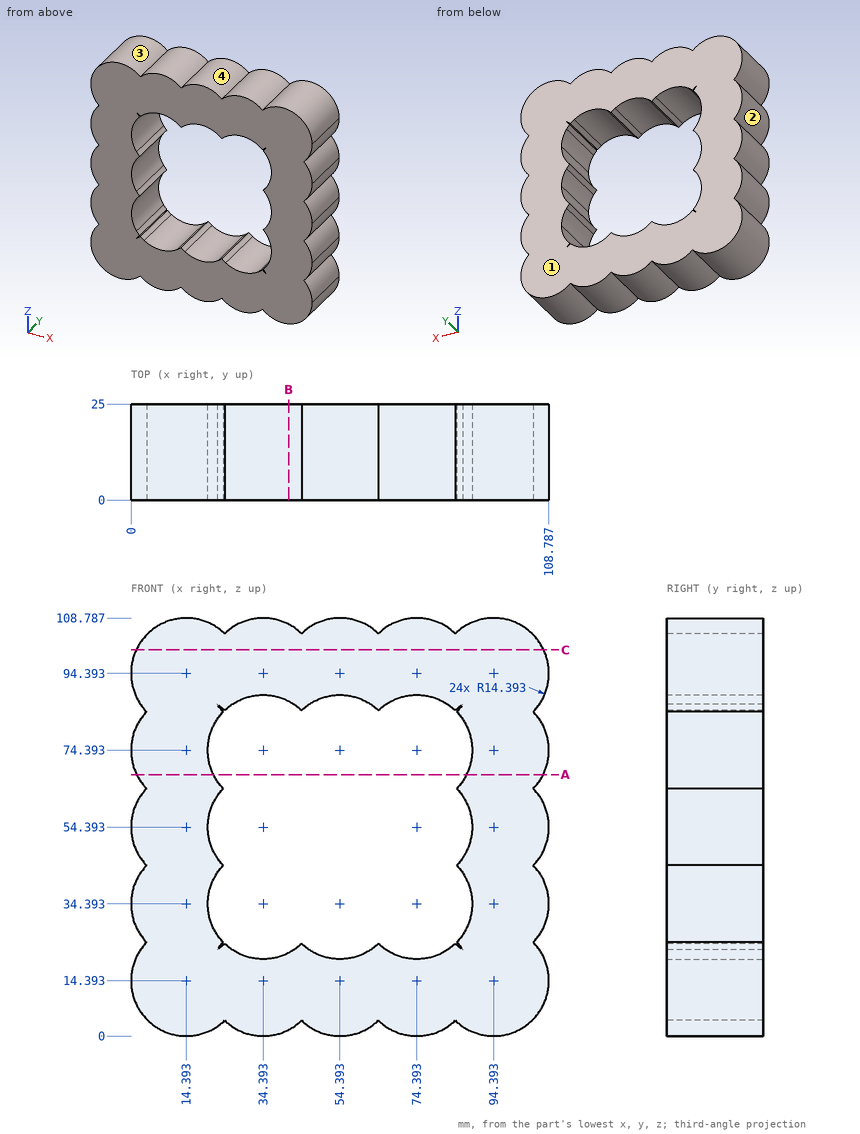
Source: three-view drawing plus pictorial views. Frame: mm from the lowest corner of the part. Give positions to 0.01 mm unless a question says otherwise; leave off trailing zeros. Write each loop counter-clockwise with the first axis right and the second up, starting at its lowest first coordinate (ties: lowest second). Pieces come first, ordered by that corner, then holes. Notation, with made-up numbers: (56.25, 68.5) -> (63.25, 68.5) arc R32 ccw to (63.25, 101.5) -> close; hole circle Ø8 at (-7, 42.5). An arc over 180 degrees is marked (long way). Answer in a Markdown table with one row per item.
(1) Draft query along Z for the marked faces 1, 2, 3 and 4. Return one class per face: +Z half, -Z half, draft (parallel to the pull), parting line (faces both ways), or undercut.
Answers below:
| item | result |
|---|---|
| face 1 | draft |
| face 2 | undercut |
| face 3 | undercut |
| face 4 | +Z half |
(2) Section query B-B on x = 41. Return loops of the section in (y, z), then the cut area to 4 significant figures.
Answers below:
| item | result |
|---|---|
| outline | (0, 1.61) -> (25, 1.61) -> (25, 21.61) -> (0, 21.61) -> close; (0, 87.18) -> (25, 87.18) -> (25, 107.18) -> (0, 107.18) -> close |
| area | 1,000 mm^2 |
(3) Section query A-A on z = 68. Return loops of the section in (x, y), then the cut area to 4 significant figures.
Answers below:
| item | result |
|---|---|
| outline | (1.5, 0) -> (21.5, 0) -> (21.5, 25) -> (1.5, 25) -> close; (87.29, 0) -> (107.29, 0) -> (107.29, 25) -> (87.29, 25) -> close |
| area | 1,000 mm^2 |
(4) Pin query (flat end, axial travel): pin 1 (6 mm diameter, centred on y = 8.5, z = 24, fed in from +X); pin 2 (5 mm diameter, centred on x = 94, y = 6.5, fed in from -Z); pin 3 (2 mm diameter, centred on x = 65.5, y = 6, fed in from -Z); pin 4 (3 mm diameter, centred on y = 8.5, z = 11.5, fed in from +X). Return the tip coordinate at first contact, or that it passes through.
Answers below:
| item | result |
|---|---|
| pin 1 | x = 107.18 |
| pin 2 | z = 0 |
| pin 3 | z = 2.36 |
| pin 4 | x = 108.72 |
(5) Section query C-C on z = 100.5. Return loops of the section in (x, y), then the cut area to 3 significant figures.
Answers below:
| item | result |
|---|---|
| outline | (1.36, 0) -> (107.43, 0) -> (107.43, 25) -> (1.36, 25) -> close |
| area | 2,650 mm^2 |
(6) Ray query, line 1 along Z through (x, y) = (86, 13) (1 decimal); line 2 along X through (y, z) = (23, 87.5) (1 decimal); line 3 along X through (y, z) = (17.5, 25). Return the intervals inside material, ascending. Write a range as [from, to].
Answers below:
| item | result |
|---|---|
| line 1 | [2.7, 22.7], [22.9, 25.9], [42.9, 45.9], [62.9, 65.9], [82.9, 85.9], [86.1, 106.1] |
| line 2 | [1.8, 28.4], [40.3, 48.4], [60.3, 68.4], [80.3, 107] |
| line 3 | [3.49, 23.49], [85.3, 105.3] |
